Can you work these out from the drawing? Everything is in mm from the part's minimum corner. Give positions to 0.01 mm unless a question says otherwise; leave off trailing zeros. Write each loop counter-clockwise with the first axis right and the second up, starting at its lowest first coordinate (ties: lowest second). Pieces come first, ordered by that corner, then holes. Notation, with made-up numbers: (35, 5.5) -> (89, 5.5) arc R28 cw to (89, 40.5) -> close; hole circle Ø2 at (-22.75, 25). An arc over 180 degrees is marked (long way). Return JSON: item names as keys, results as strings.
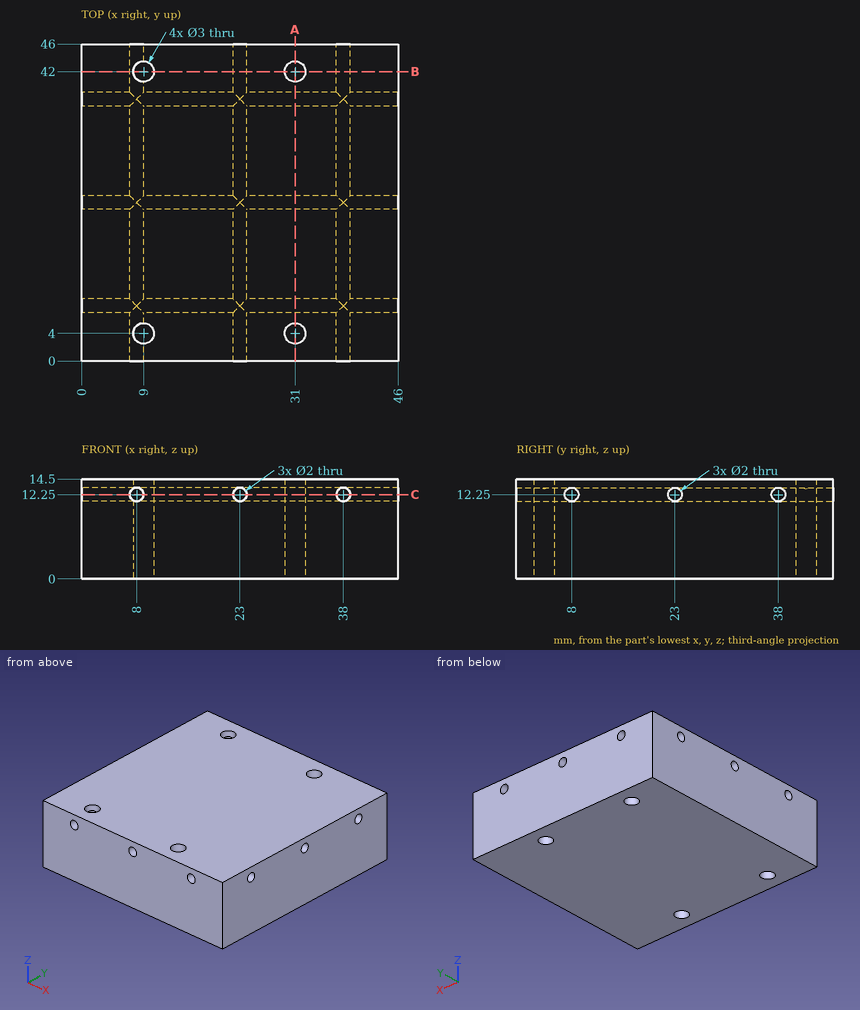
1. Suppose I cut it at A-A, the plane x = 31. List the corners of the cut face in (y, z) for me, and give its area (3 significant figures).
Taken from the geometry:
{"outline": "(0, 0) -> (2.5, 0) -> (2.5, 14.5) -> (0, 14.5) -> close; (5.5, 0) -> (40.5, 0) -> (40.5, 14.5) -> (5.5, 14.5) -> close; (43.5, 0) -> (46, 0) -> (46, 14.5) -> (43.5, 14.5) -> close; hole circle Ø2 at (8, 12.25); hole circle Ø2 at (23, 12.25); hole circle Ø2 at (38, 12.25)", "area": "571 mm²"}
2. If I drill on line 1 (Z direction, x = 23, y = 26.75); line 2 (X direction, y = 27.5, z = 12.5); line 3 (Y direction, x = 32, z = 2.75), over which ranges is the centre line in solid material (lowest first)? Write a range as [from, to].
Taken from the geometry:
{"line 1": "z = [0, 11.25], [13.25, 14.5]", "line 2": "x = [0, 7.03], [8.97, 22.03], [23.97, 37.03], [38.97, 46]", "line 3": "y = [0, 2.88], [5.12, 40.88], [43.12, 46]"}
3. Suppose I cut it at B-B, the plane y = 42. List the corners of the cut face in (x, z) for me.
Taken from the geometry:
{"outline": "(0, 0) -> (7.5, 0) -> (7.5, 11.38) arc R1 cw to (7.5, 13.12) -> (7.5, 14.5) -> (0, 14.5) -> close; (10.5, 0) -> (29.5, 0) -> (29.5, 14.5) -> (10.5, 14.5) -> close; (32.5, 0) -> (46, 0) -> (46, 14.5) -> (32.5, 14.5) -> close; hole circle Ø2 at (23, 12.25); hole circle Ø2 at (38, 12.25)"}
4. Suppose I cut it at C-C, the plane z = 12.25. Count the separate pieces of the cut face and the enclosed holes in it, and give its area (3 significant figures).
Taken from the geometry:
{"separate pieces": "16", "enclosed holes": "2", "area": "1,580 mm²"}
5. For pin 1 Ø2.5 at (y, z) = (23, 12.25) entering from -X, with a flat end and sliding along its axis, tell me the tip position at first contact or that it passes through.
Taken from the geometry:
{"pin 1": "stops at x = 0"}
